For this review, take the finished solid that the model builds, in its own axes (mm). Coordinates: 2 decimals unless noted, no trailing zeros. Loops run counter-clockwise (first coordinate to the right, second up) from the corner with the lowest first, then second, coordinate; pieces in that order, holes last. Notation, with made-up numbers: M 65.25,-6 L 119.25,-6 A28 ccw 119.25,13 Z; hole C 47.25,17 d11. An arc over 180 degrees is marked long. Answer as a JSON object with one key per item and string values. Group by question number.
Item 1: Add section A-A (y = 63). State the section outline as (x, z) points.
Item 2: Add section B-B (z = 27.45). Count the separate pieces of the cut face and the enclosed holes in it, then the cut area to 3 significant figures.
Item 3: Wall thickness on L1, parallel to Y at x = 255, z = 27.35; L2, parallel to X at y = 255, z = 26.75; L3, parallel to X at y = 81.5, z = 26.85: over which ranges is each line inside the solid? List them lowest first. Write a range as from..to.
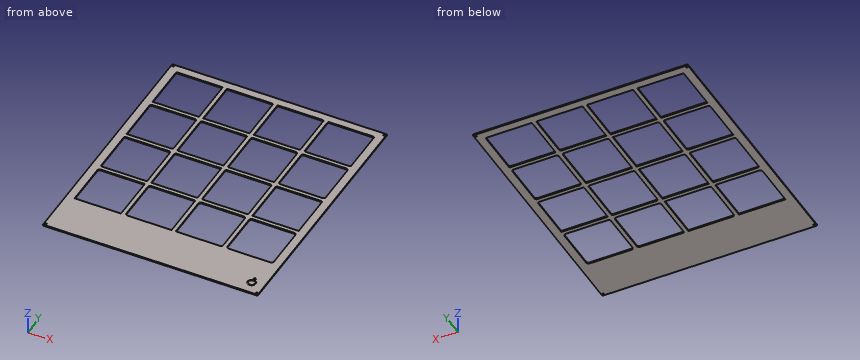
from build123d import *

# Parameters (mm, degrees)
SKETCH_W            = 520
SKETCH_H            = 610
PAD_DEPTH           = 3
SKETCH001_W         = 112.5
SKETCH001_H         = 112.5
POCKET_DEPTH        = 3.001
LINEARPATTERN_COUNT = 4
LINEARPATTERN_PITCH = 122.5
FILLET_R            = 3
FILLET001_R         = 4
FILLET002_R         = 5
FILLET003_R         = 6
SKETCH002_R         = 1.6
POCKET001_DEPTH     = 5
SKETCH003_R         = 10
SKETCH003_R_2       = 7
POCKET002_DEPTH     = 1.2


with BuildPart() as part:
    # Sketch → Pad (new body)
    with BuildSketch(Plane.XY):
        with Locations((0, -45)):
            Rectangle(SKETCH_W, SKETCH_H)
    extrude(amount=-PAD_DEPTH)

    # Sketch001 (on Face5 of Pad) → Pocket (cut, through all)
    with BuildSketch(Plane.XY):
        with Locations((-183.75, 183.75)):
            Rectangle(SKETCH001_W, SKETCH001_H)
        with Locations((-61.25, 183.75)):
            Rectangle(SKETCH001_W, SKETCH001_H)
        with Locations((61.25, 183.75)):
            Rectangle(SKETCH001_W, SKETCH001_H)
        with Locations((183.75, 183.75)):
            Rectangle(SKETCH001_W, SKETCH001_H)
    pocket = extrude(amount=-POCKET_DEPTH, mode=Mode.SUBTRACT)

    # LinearPattern: Pocket ×4
    with Locations(*[(0, -i * LINEARPATTERN_PITCH, 0) for i in range(1, LINEARPATTERN_COUNT)]):
        add(pocket, mode=Mode.SUBTRACT)

    # Fillet
    fillet_edges = [part.edges().sort_by_distance(p)[0] for p in [
        (-240, 240, -1.5),
        (-117.5, 240, -1.5),
        (-5, 240, -1.5),
        (5, 240, -1.5),
        (117.5, 240, -1.5),
        (117.5, 127.5, -1.5),
        (240, 127.5, -1.5),
        (240, 240, -1.5),
        (127.5, 240, -1.5),
        (127.5, 127.5, -1.5),
    ]]
    fillet(fillet_edges, radius=FILLET_R)

    # Fillet001
    fillet001_edges = [part.edges().sort_by_distance(p)[0] for p in [
        (-117.5, 117.5, -1.5),
        (127.5, -5, -1.5),
        (240, -5, -1.5),
        (-240, -117.5, -1.5),
        (-240, -5, -1.5),
        (-127.5, -5, -1.5),
        (117.5, -5, -1.5),
        (117.5, -117.5, -1.5),
        (5, -117.5, -1.5),
        (5, -5, -1.5),
    ]]
    fillet(fillet001_edges, radius=FILLET001_R)

    # Fillet002
    fillet002_edges = [part.edges().sort_by_distance(p)[0] for p in [
        (-117.5, -5, -1.5),
        (5, 117.5, -1.5),
        (117.5, 117.5, -1.5),
        (-240, 117.5, -1.5),
        (-127.5, 117.5, -1.5),
        (-127.5, 5, -1.5),
        (240, 5, -1.5),
        (127.5, 5, -1.5),
        (127.5, 117.5, -1.5),
        (240, 117.5, -1.5),
    ]]
    fillet(fillet002_edges, radius=FILLET002_R)

    # Fillet003
    fillet003_edges = [part.edges().sort_by_distance(p)[0] for p in [
        (-240, -127.5, -1.5),
        (-117.5, -127.5, -1.5),
        (-117.5, -240, -1.5),
        (5, -127.5, -1.5),
        (117.5, -127.5, -1.5),
        (117.5, -240, -1.5),
        (127.5, -127.5, -1.5),
        (240, -127.5, -1.5),
        (240, -240, -1.5),
        (127.5, -240, -1.5),
    ]]
    fillet(fillet003_edges, radius=FILLET003_R)

    # Sketch002 (on Face1 of Fillet003) → Pocket001 (cut)
    with BuildSketch(Plane.XY):
        with Locations((-255, 255)):
            Circle(SKETCH002_R)
        with Locations((255, 255)):
            Circle(SKETCH002_R)
        with Locations((255, -345)):
            Circle(SKETCH002_R)
        with Locations((-255, -345)):
            Circle(SKETCH002_R)
    extrude(amount=-POCKET001_DEPTH, mode=Mode.SUBTRACT)

    # Sketch003 (on Face1 of Pocket001) → Pocket002 (cut)
    with BuildSketch(Plane.XY):
        with Locations((230, -320)):
            Circle(SKETCH003_R)
        with Locations((230, -320)):
            Circle(SKETCH003_R_2, mode=Mode.SUBTRACT)
        Polygon((230, -301), (226.535898, -307), (233.464102, -307), align=None)
    extrude(amount=-POCKET002_DEPTH, mode=Mode.SUBTRACT)


with BuildPart() as part_1:
    # Body placement: moved
    add(part.part.moved(Location((0, 0, 28))))


solid = part_1.part
From the geometry:
{
 "1": {"outline": "M -260,25 L -240,25 L -240,28 L -260,28 Z; M -127.5,25 L -117.5,25 L -117.5,28 L -127.5,28 Z; M -5,25 L 5,25 L 5,28 L -5,28 Z; M 117.5,25 L 127.5,25 L 127.5,28 L 117.5,28 Z; M 240,25 L 260,25 L 260,28 L 240,28 Z"},
 "2": {"separate pieces": "2", "enclosed holes": "22", "area": "115,000 mm²"},
 "3": {"L1": "y = -350..-346.6, -343.4..253.4, 256.6..260", "L2": "x = -260..-256.6, -253.4..253.4, 256.6..260", "L3": "x = -260..-240, -127.5..-117.5, -5..5, 117.5..127.5, 240..260"}
}
